CAD build for the part. Positions are in the model's coordinates, mm. A direction names the side the tool comes from. Give positions to 0.01 mm unless a question says otherwise; leave off trailing zeros. Write each loop counter-clockwise with the first axis right and the second up, starting at its lowest first coordinate (ties: lowest second). Pieces come first, ordered by that corner, then holes. Notation, with made-up numbers: (83, 23.5) - (119, 23.5) arc R26 cw to (119, 48.5) - close; hole circle Ø10 at (4.25, -37). An arc over 180 degrees is marked (long way). Answer as a JSON object with one key per item and string values.
from build123d import *

# Parameters (mm, degrees)
CUT_EXTRUDE_3_DEPTH    = 11.5
HOLE_WIZARD_M3_1_D     = 2.5
HOLE_WIZARD_M3_1_DEPTH = 8
HOLE_WIZARD_M3_1_TIP   = 0.751075774
SKETCH_12_R            = 1.5
CUT_EXTRUDE_4_DEPTH    = 11.5
HOLE_WIZARD_M3_2_D     = 2.5
HOLE_WIZARD_M3_2_DEPTH = 4
HOLE_WIZARD_M3_2_TIP   = 0.751075774
EXTRUDE_1_DEPTH        = 0.5


with BuildPart() as part:
    # 草图1 → 旋转1 (revolve)
    with BuildSketch(Plane(origin=(0, 0, 0), x_dir=(1, 0, 0), z_dir=(0, 1, 0))):
        Polygon((0, 0), (-29, 0), (-29, 5.7), (-31.6, 5.7), (-31.6, 9.2), (-46, 9.2), (-46, 12.2), (0, 12.2), align=None)
    revolve(axis=Axis((-46, 0, -12.2), (1, 0, 0)))

    # 草图9 → 切除-拉伸3 (cut)
    with BuildSketch(Plane.ZY.offset(46)):
        with BuildLine():
            Line((-12.2, 2.5), (-10.541687605, 2.5))
            ThreePointArc((-10.541687605, 2.5), (-12.2, 3), (-13.858312395, 2.5))
            Line((-13.858312395, 2.5), (-12.2, 2.5))
        make_face()
    extrude(amount=-CUT_EXTRUDE_3_DEPTH, mode=Mode.SUBTRACT)

    # M3 螺纹孔1
    with Locations(Plane.ZY.offset(46)):
        with Locations((-12.2, 0)):
            Hole(HOLE_WIZARD_M3_1_D / 2, depth=HOLE_WIZARD_M3_1_DEPTH)
            with Locations((0, 0, -(HOLE_WIZARD_M3_1_DEPTH + HOLE_WIZARD_M3_1_TIP / 2))):  # 118° drill point
                Cone(0, HOLE_WIZARD_M3_1_D / 2, HOLE_WIZARD_M3_1_TIP, mode=Mode.SUBTRACT)

    # 草图12 → 切除-拉伸4 (cut)
    with BuildSketch(Plane(origin=(0, 2.5, 0), x_dir=(1, 0, 0), z_dir=(0, 1, 0))):
        with Locations((-37, 12.2)):
            Circle(SKETCH_12_R)
    extrude(amount=-CUT_EXTRUDE_4_DEPTH, mode=Mode.SUBTRACT)

    # M3 螺纹孔2
    with Locations(Plane.ZY.offset(29)):
        with Locations((-12.2, 9.5), (-20.427241336, -4.75), (-3.972758664, -4.75)):
            Hole(HOLE_WIZARD_M3_2_D / 2, depth=HOLE_WIZARD_M3_2_DEPTH)
            with Locations((0, 0, -(HOLE_WIZARD_M3_2_DEPTH + HOLE_WIZARD_M3_2_TIP / 2))):  # 118° drill point
                Cone(0, HOLE_WIZARD_M3_2_D / 2, HOLE_WIZARD_M3_2_TIP, mode=Mode.SUBTRACT)

    # 草图16 → 凸台-拉伸1 (add)
    with BuildSketch(Plane.ZY.offset(31.6)):
        with BuildLine():
            Line((-9.601923789, -1.5), (-12.2, -6))
            ThreePointArc((-12.2, -6), (-8.525765386, 4.74341649), (-18.009475019, -1.5))
            Line((-18.009475019, -1.5), (-14.69206472, 1.670213589))
            ThreePointArc((-14.69206472, 1.670213589), (-10.614007201, 2.546493048), (-9.601923789, -1.5))
        make_face()
    extrude(amount=EXTRUDE_1_DEPTH)


solid = part.part
Item 1: Probe line 1 (Y direction, x = -40, z = -12.2); line 2 (Z direction, x = -40.5, y = 0); line 3 (Z direction, x = -27.7, y = -4.75). List the from-to ranges inside material, lowest first. Write a range as from..to.
Entries:
{"line 1": "-3..-1.25, 1.25..2.5", "line 2": "-15.2..-13.45, -10.95..-9.2", "line 3": "-23.44..-21.68, -19.18..-5.22, -2.72..-0.96"}
Item 2: Which spindle directions (+Z, -Z, +X, -X, +Y, -Y) get a long thin tool onto all of the face, cutting with end or side? Do faces 1 (the cylindrical face through (-14.703, -12.096, -13.788)), 2 (the flat face through (-42, 2.5, -12)), 3 (the cylindrical face through (-31.85, 4.61, -8.36)). Say none if no direction does.
Entries:
{"face 1": "+X, -X", "face 2": "+Z, -Z, -X, +Y", "face 3": "-X"}
Item 3: Flat gauge pins, fed straight in: P1, Ø1.5, axis at x = -5, z = -15.5, coming from the +Y side; P2, Ø4, axis at y = 9.5, z = -12.2, coming from the -X side; P3, Ø2, axis at y = 0, z = -12.2, coming from the -X side. Where does each tip first touch, or does it go through?
Entries:
{"P1": "y = 11.93", "P2": "x = -29", "P3": "x = -35.88"}
Item 4: Cut at C-C (z = -7.5). Give the cut face in (x, y), and give its area (3 significant figures).
Entries:
{"outline": "(-32.1, -3.73) - (-31.6, -3.73) - (-31.6, -4.49) - (-29, -4.49) - (-29, -11.26) - (0, -11.26) - (0, 11.26) - (-29, 11.26) - (-29, 4.49) - (-31.6, 4.49) - (-31.6, 3.73) - (-32.1, 3.73) - close", "area": "680 mm2"}
Item 5: Cut at D-D (x = -12.5). Give the cut face in (y, z).
Entries:
{"outline": "circle Ø24.4 at (0, -12.2)"}
Item 6: Mould opens along Z. For faces 4 (the flat face through (0, 0, -12)), 5 (the cylindrical face through (-26.97, -5.86, -4.55)), 6 (the cylindrical face through (-30.318, -0.286, -18.694)) say: +Z half, -Z half, draft (parallel to the pull), parting line (faces both ways), or undercut.
Entries:
{"face 4": "draft", "face 5": "undercut", "face 6": "parting line"}
Item 7: Cut at A-A (y = 0). Give the cut face in (x, z).
Entries:
{"outline": "(-46, -15.2) - (-31.6, -15.2) - (-31.6, -16.44) - (-32.1, -16.44) - (-32.1, -18.2) - (-31.6, -18.2) - (-31.6, -18.7) - (-29, -18.7) - (-29, -24.4) - (0, -24.4) - (0, 0) - (-29, 0) - (-29, -5.7) - (-31.6, -5.7) - (-31.6, -6.2) - (-32.1, -6.2) - (-32.1, -9.2) - (-46, -9.2) - (-46, -10.95) - (-38, -10.95) - (-37.95, -11.04) arc R1.5 cw (long way) to (-37.95, -13.36) - (-38, -13.45) - (-46, -13.45) - close"}
Item 8: Cut at B-B (x = -37). Give the cut face in (y, z), and give its area (3 significant figures).
Entries:
{"outline": "(-2.6, -13.7) arc R3 ccw to (2.5, -13.86) - (2.5, -13.7) - close; (-2.6, -10.7) - (2.5, -10.7) - (2.5, -10.54) arc R3 ccw to start", "area": "11.0 mm2"}
